Input: dimensioned drawing with shaded views. Units: mm. Origin: part minimum x, y, z. A direction names the side the tool comes from. Give positions to 0.01 mm unless a question says otherwise; leave off trailing zeros. Answer in a Markdown table with one row per item. Add a question column.
1) Section query D-D (y = 1.9). Give the number of separate pieces and of enclosed holes in the cut face.
2) Access query for the marked faces 1, 2, 3, 4 and 5. Directions: +Z, -Z, +X, -X, +Y, -Y. A direction counts if a zero-diameter tool reaches every point of the face in a straight line with its end or side. Return the directions, or none.
3) Line query: line 1 (Z direction, x = 3.5, y = 0.2) (1 decimal); line 2 (Z direction, x = 2.5, y = 2.6); line 3 (X direction, y = 1.9, z = 11). Output: solid intervals per line, ascending. Write a range as from..to.
4) First-contact query: P1, Ø1.6, axis at x = 4.5, y = 1.5, coming from the -Z side; P2, Ø1, axis at y = 2, z = 10, coming from the -X side; P3, Ø1.5, axis at x = 1, y = 1.5, coming from the +Z side. Flat tips, straight axial feed; report the tip coordinate or a pass-through.
5) Draft query along Z for the marked faces 6, 7 and 8. Return one class per face: +Z half, -Z half, draft (parallel to the pull), parting line (faces both ways), or undercut.
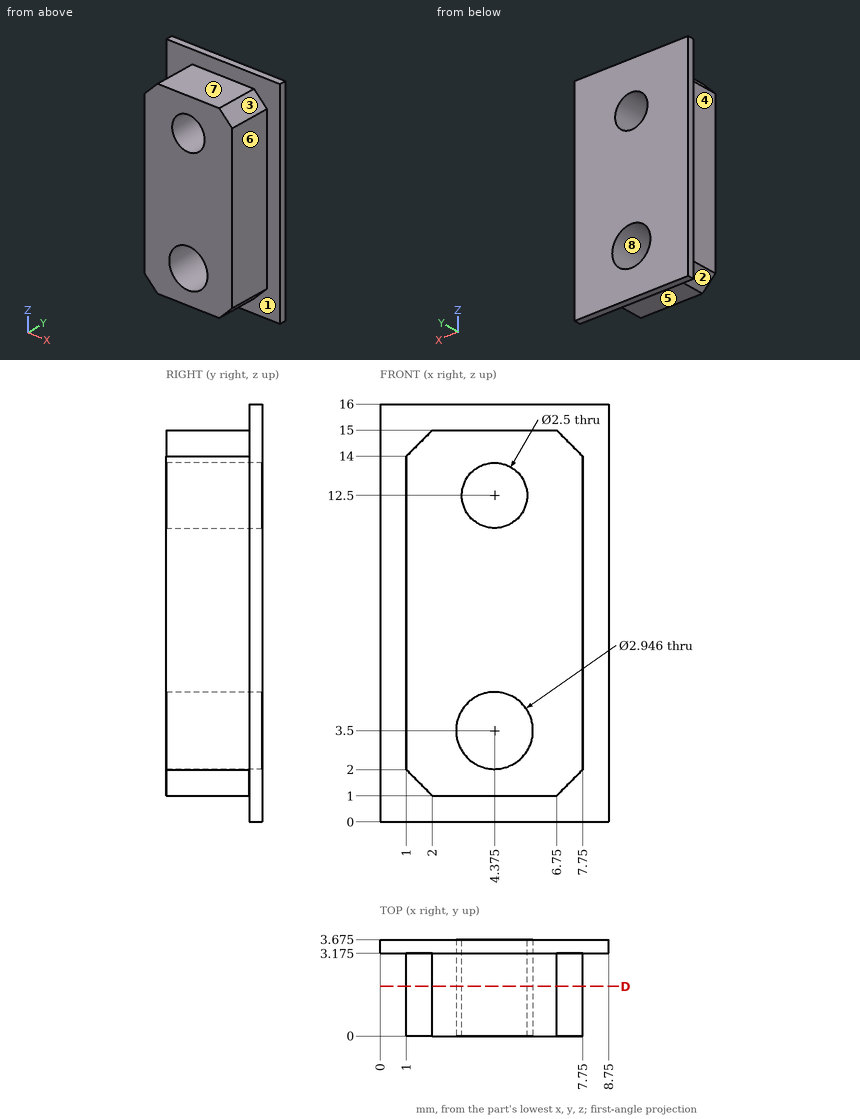
Evaluation:
| question | item | result |
|---|---|---|
| 1 | separate pieces | 1 |
| 1 | enclosed holes | 2 |
| 2 | face 1 | -Y |
| 2 | face 2 | -Z, -X, -Y |
| 2 | face 3 | +Z, +X, -Y |
| 2 | face 4 | +Z, -Z, -X, -Y |
| 2 | face 5 | -Z, +X, -X, -Y |
| 3 | line 1 | 1..2.3, 4.7..11.6, 13.4..15 |
| 3 | line 2 | 1..15 |
| 3 | line 3 | 1..7.75 |
| 4 | P1 | z = 1 |
| 4 | P2 | x = 1 |
| 4 | P3 | z = 14.75 |
| 5 | face 6 | draft |
| 5 | face 7 | +Z half |
| 5 | face 8 | undercut |
